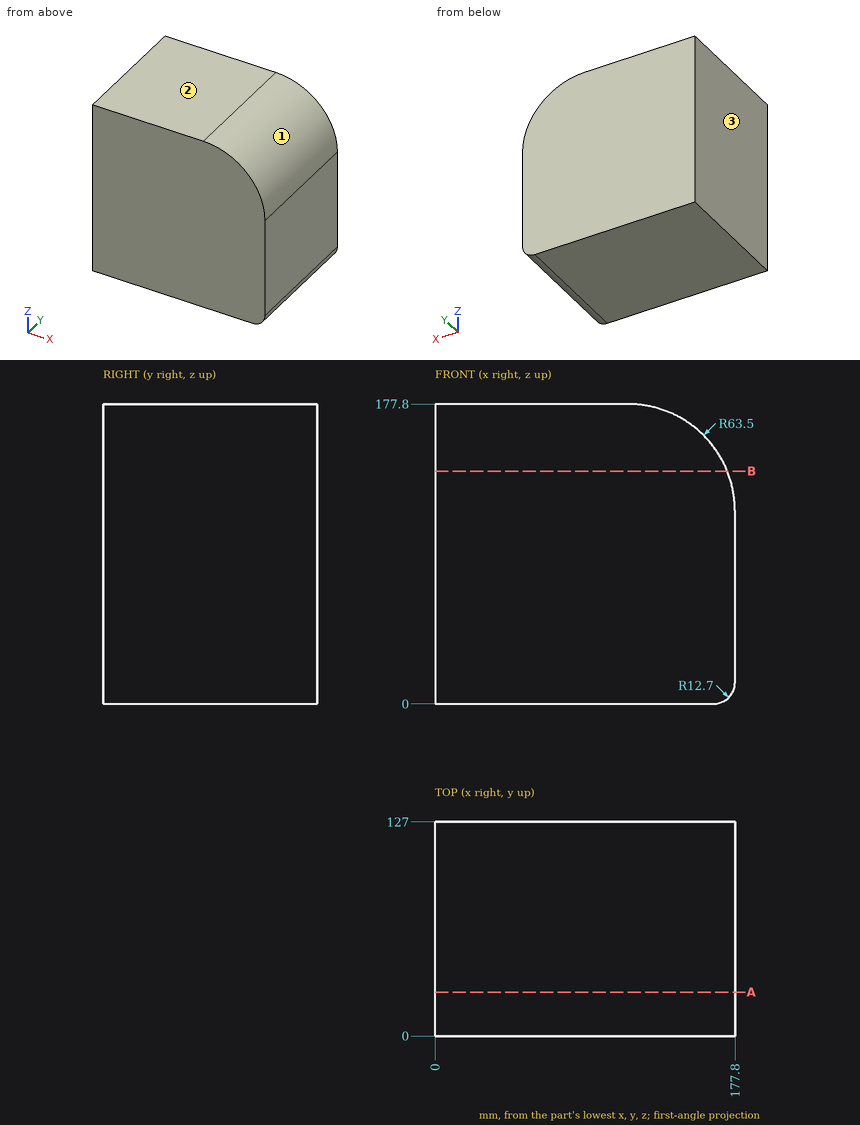
Here's the drawing with two shaded views (mm, measured from the low corner). I have some questions. Coordinates: 2 decimals unless noted, no trailing zeros. Loops run counter-clockwise (first coordinate to the right, second up) from the corner with the lowest first, then second, coordinate; pieces in that order, holes last. Notation, with made-up numbers: (60, -12) -> (78, -12) arc R11 ccw to (78, 9) -> close; hole circle Ø7 at (87.25, -29). An arc over 180 degrees is marked (long way). Put each result on its own line as item: value. Start each with the question number.
Q1. I'm going to push flat-ended pins straight in: P1, Ø1, axis at y = 32, z = 144.5, coming from the +X side; P2, Ø12, axis at x = 153.5, y = 46, coming from the +Z side; P3, Ø6, axis at x = 123, y = 112.5, coming from the +Z side. Where does each tip first touch, or does it pass through?
Q2. If I drill on line 1 (Z direction, x = 147, y = 33); line 2 (X direction, y = 24, z = 160); line 3 (X direction, y = 98, z = 122.5), over which ranges is the centre line in solid material (lowest first)? Write a range as [from, to].
Q3. I want a section at A-A (y = 26). Write out the boundary of the cut face in (x, z), plus the area to 3 significant figures.
Q4. Thinking about a two-plate mould opening in X: for the marked faces 1, 2 and 3, which applies, pulls with the +X half, pulls with the -X half, needs draft (parallel to the pull), parting line crosses it, or undercut?
Q5. I want a section at B-B (z = 138). Write out the boundary of the cut face in (x, y).
Taken from the geometry:
1. P1: stops at x = 170.43
1. P2: stops at z = 168.43
1. P3: stops at z = 177.54
2. line 1: z = [0, 168.73]
2. line 2: x = [0, 158.39]
2. line 3: x = [0, 177.27]
3. outline: (0, 0) -> (165.1, 0) arc R12.7 ccw to (177.8, 12.7) -> (177.8, 114.3) arc R63.5 ccw to (114.3, 177.8) -> (0, 177.8) -> close
3. area: 30,700 mm2
4. face 1: pulls with the +X half
4. face 2: needs draft
4. face 3: pulls with the -X half
5. outline: (0, 0) -> (173.21, 0) -> (173.21, 127) -> (0, 127) -> close
